Geometry: final body of the model. Coordinates: model frame, mm. Face numbers are marked on the shaded views. A direction names the side the tool comes from. Give positions to 0.01 mm unless a question says otherwise; leave off trailing zeros. Write each loop counter-clockwise with the first axis right and the second up, starting at its lowest first coordinate (ties: lowest second). Pieces come first, ordered by that corner, then holes.
Q1. Line query: line 1 (X direction, y = 4.05, z = -1.05); line 2 (X direction, y = 3.1, z = 0.75); line 3 (Z direction, x = 6.75, y = 3.25). Output: solid intervals per line, ascending.
Q2. Section B-B (x = 7). Return the cut outline in (y, z), plus the area to 3 significant figures.
Q3. Section A-A (z = 0). Return the cut outline in (x, y), plus the area to 3 significant figures.
Q4. Reachability of the marked faces 3 and 4 from +Z, -Z, +X, -X, +Y, -Y: full face, straight path, thin tool, end or side. Return the list, or none.
Q5. Pin query (flat end, axial travel): pin 1 Ø2 at (x, z) = (11, -1.5) entering from +Y; pin 2 Ø1.5 at (x, y) = (10, 2.5) entering from -Z. Return the tip coordinate at first contact, or that it passes through.
Q6. Mould query, pull axis Y, two halves, no side actions, for the marked faces 1 and 2. Classes: +Y half, -Y half, draft (parallel to the pull), parting line (faces both ways), or undercut.
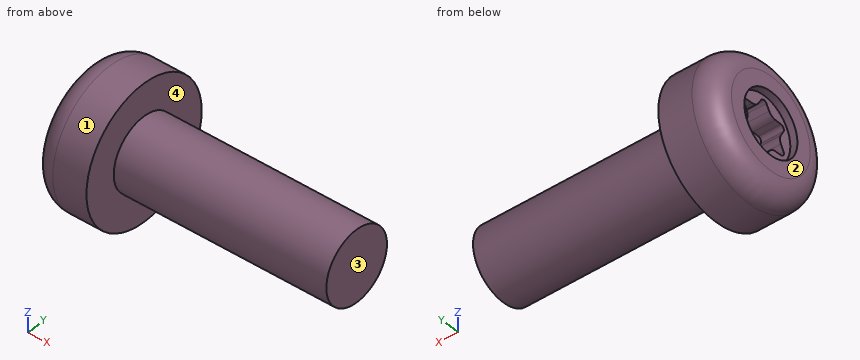
from build123d import *

# Parameters (mm, degrees)
F0_W     = 1.55
F0_H     = 1.9
F2_R     = 0.6
F3_R     = 0.875
F4_DEPTH = 0.2
F5_R     = 1
F6_DEPTH = 6
F8_DEPTH = 0.64
F9_R     = 0.1
F10_R    = 0.25


with BuildPart() as f1:
    # F0 (on Top) → F1 (revolve)
    with BuildSketch(Plane.XY):
        with Locations((5.8241569564, 4.3333681053)):
            Rectangle(F0_W, F0_H)
    revolve(axis=Axis((5.8241569564, 3.3833681053, 0), (-1, 0, 0)))

    # F2
    f2_edges = [f1.edges().sort_by_distance(p)[0] for p in [
        (5.049157, 1.483368, 0),
    ]]
    fillet(f2_edges, radius=F2_R)

    # F3 (on face) → F4 (cut)
    with BuildSketch(Plane(origin=(5.0491569564, 0, 0), x_dir=(0, -1, 0), z_dir=(-1, 0, 0))):
        with Locations((-3.3833681053, 0)):
            Circle(F3_R)
    extrude(amount=-F4_DEPTH, mode=Mode.SUBTRACT)

    # F5 (on face) → F6 (join)
    with BuildSketch(Plane.YZ.offset(6.5991569564)):
        with Locations((3.3833681053, 0)):
            Circle(F5_R)
    extrude(amount=F6_DEPTH)

    # F7 (on face) → F8 (cut)
    with BuildSketch(Plane(origin=(5.2491569564, 0, 0), x_dir=(0, -1, 0), z_dir=(-1, 0, 0))):
        Polygon((-3.1333681053, 0.4330127019), (-3.3833681053, 0.84), (-3.6333681053, 0.4330127019), (-4.1108294444, 0.42), (-3.8833681053, 0), (-4.1108294444, -0.42), (-3.6333681053, -0.4330127019), (-3.3833681053, -0.84), (-3.1333681053, -0.4330127019), (-2.6559067661, -0.42), (-2.8833681053, 0), (-2.6559067661, 0.42), align=None)
    extrude(amount=-F8_DEPTH, mode=Mode.SUBTRACT)

    # F9
    f9_edges = [f1.edges().sort_by_distance(p)[0] for p in [
        (5.569157, 3.383368, 0.84),
        (5.569157, 4.110829, 0.42),
        (5.569157, 4.110829, -0.42),
        (5.569157, 3.383368, -0.84),
        (5.569157, 2.655907, -0.42),
        (5.569157, 2.655907, 0.42),
    ]]
    fillet(f9_edges, radius=F9_R)

    # F10
    f10_edges = [f1.edges().sort_by_distance(p)[0] for p in [
        (5.569157, 3.633368, 0.433013),
        (5.569157, 3.883368, 0),
        (5.569157, 3.633368, -0.433013),
        (5.569157, 3.133368, 0.433013),
        (5.569157, 3.133368, -0.433013),
        (5.569157, 2.883368, 0),
    ]]
    fillet(f10_edges, radius=F10_R)


solid = f1.part
Computed:
1. line 1: x = 5.05 to 6.6
1. line 2: x = 5.25 to 12.6
1. line 3: z = -0.99 to 0.99
2. outline: circle Ø2 at (3.38, 0)
2. area: 3.14 mm2
3. outline: (5.05, 2.08) arc R0.6 ccw to (5.65, 1.48) - (6.6, 1.48) - (6.6, 2.38) - (12.6, 2.38) - (12.6, 4.38) - (6.6, 4.38) - (6.6, 5.28) - (5.65, 5.28) arc R0.6 ccw to (5.05, 4.68) - (5.05, 4.26) - (5.25, 4.26) - (5.25, 3.92) - (5.89, 3.92) - (5.89, 2.85) - (5.25, 2.85) - (5.25, 2.51) - (5.05, 2.51) - close
3. area: 16.7 mm2
4. face 3: +Z, -Z, +X, +Y, -Y
4. face 4: +X
5. pin 1: stops at y = 4.25
5. pin 2: stops at z = -0.99
6. face 1: parting line
6. face 2: draft
